Autodesk Inventor part; units mm, degrees
ref_plane "YZ Plane" through (0, 0, 0) normal (1, 0, 0) x (0, 1, 0)
ref_plane "XZ Plane" through (0, 0, 0) normal (0, 1, 0) x (-1, 0, 0)
ref_plane "XY Plane" through (0, 0, 0) normal (0, 0, 1) x (1, 0, 0)
sketch "Sketch1" plane through (0, 0, 0) normal (0, 0, 1) x (1, 0, 0)
  line L0 (0, 0) -> (60, 0)
  line L1 (60, 0) -> (60, 40)
  line L2 (60, 40) -> (0, 40)
  line L3 (0, 40) -> (0, 0)
extrude "Extrusion1" add sketch "Sketch1" along normal blind 10
sketch "Sketch2" plane through (0, 0, 0) normal (0, 0, 1) x (1, 0, 0)
  line L0 (7, 7) -> (13, 7)
  line L1 (13, 7) -> (13, 13)
  line L2 (13, 13) -> (7, 13)
  line L3 (7, 13) -> (7, 7)
extrude "Extrusion2" cut sketch "Sketch2" along normal blind 10
pattern_linear "Rectangular Pattern1" count 3 spacing 15 along (1, 0, 0) of "Extrusion2"
properties part number "21_pocket_rect"
Part model, mm, in its own coordinate system. A direction names the side the tool comes from. Round coordinates to 2 decimals unless told otherwise and drop trailing zeros. Order: outer loops, then holes, each group sorted by start corner. A loop starts at its lowest first (then second) coordinate and runs counter-clockwise, first axis right, second up. Notation, with made-up numbers: (8, -12) -> (21, -12) arc R26 cw to (21, 6) -> close; hole circle Ø1 at (63, 24). An arc over 180 degrees is marked (long way). Put each result on its own line as item: value.
Q1. Wall check: line 1 (X direction, y = 12, z = 3); line 2 (Y direction, x = 27, z = 3). Give the ranges that are in metal, low to high. Write a range as [from, to].
From the geometry:
line 1: x = [0, 7], [13, 22], [28, 37], [43, 60]
line 2: y = [0, 7], [13, 40]
Q2. Band-saw the part on B-B (z = 9.25). Give the cut face in (x, y), and give its area (3 significant figures).
From the geometry:
outline: (0, 0) -> (60, 0) -> (60, 40) -> (0, 40) -> close; hole (7, 7) -> (13, 7) -> (13, 13) -> (7, 13) -> close; hole (22, 7) -> (28, 7) -> (28, 13) -> (22, 13) -> close; hole (37, 7) -> (43, 7) -> (43, 13) -> (37, 13) -> close
area: 2,290 mm2
Q3. Pull direction X, two halves, no side cores. Call faces 3 (the face through (13, 10, 5)), 4 (the face through (60, 20, 5)), 5 (the face through (40, 7, 5)), 6 (the face through (0, 20, 5)): pulls with the +X half, pulls with the -X half, needs draft (parallel to the pull), parting line crosses it, or undercut.
From the geometry:
face 3: undercut
face 4: pulls with the +X half
face 5: undercut
face 6: pulls with the -X half
Q4. Band-saw the part on A-A (x = 10.5). Give the cut face in (y, z), and give its area (3 significant figures).
From the geometry:
outline: (0, 0) -> (7, 0) -> (7, 10) -> (0, 10) -> close; (13, 0) -> (40, 0) -> (40, 10) -> (13, 10) -> close
area: 340 mm2
Q5. Tool access for faces 1 (the face through (30, 40, 5)), 2 (the face through (7, 10, 5)): list every direction of +Z, -Z, +X, -X, +Y, -Y with a clear straight run to the whole face (end or side of a thin tool).
From the geometry:
face 1: +Z, -Z, +X, -X, +Y
face 2: +Z, -Z
